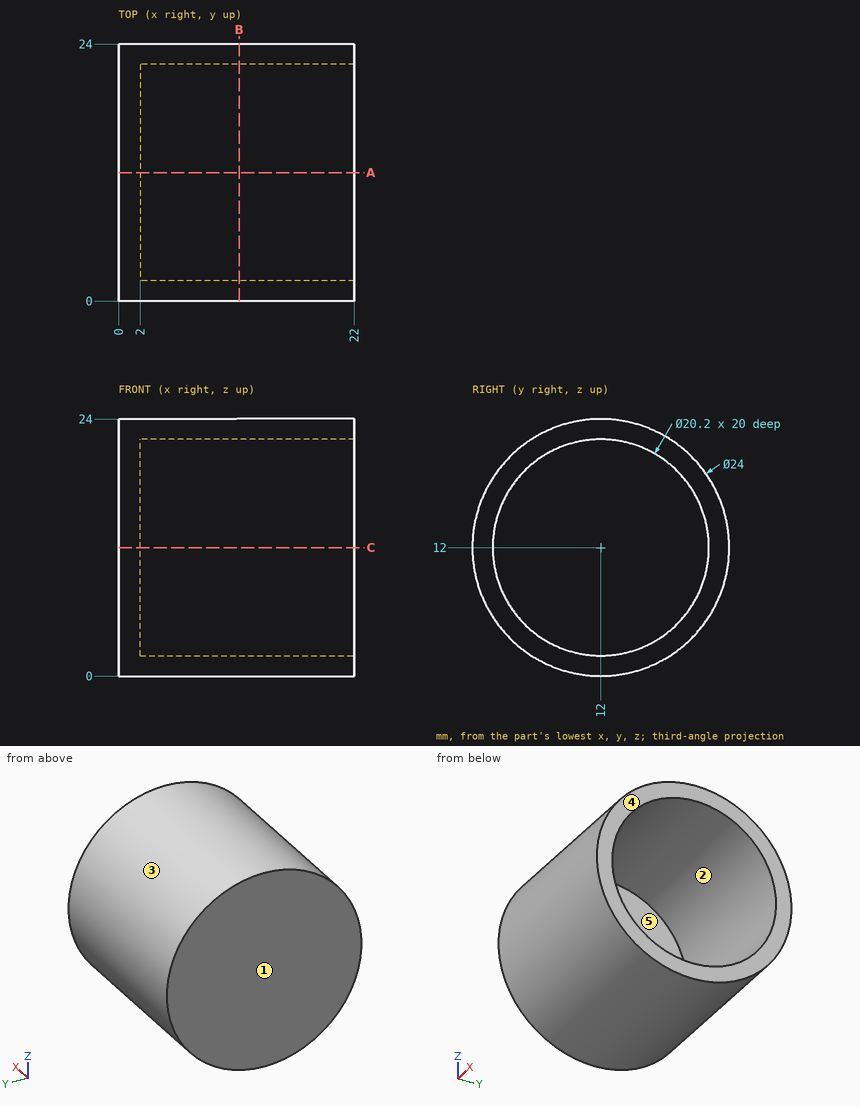
Print and shaded views of the part. All mm, measured from the part's lowest x, y and z. A direction names the side the tool comes from. Coordinates: 2 decimals unless noted, no trailing zeros. Order: outer loops, then holes, each group sorted by start corner. A loop starts at its lowest first (then second) coordinate and runs counter-clockwise, first axis right, second up. Notation, with made-up numbers: (-2, 30.25) - (48, 30.25) arc R13 cw to (48, 50.25) - close; hole circle Ø6 at (55, 46.25). An arc over 180 degrees is marked (long way). Return JSON: item names as keys, results as strings. Group by question number.
Item 1: Pull direction Y, two halves, no side cores. Call the marked faces 3, 4 and 5: pulls with the +Y half, pulls with the -Y half, needs draft (parallel to the pull), parting line crosses it, or undercut.
Item 2: Pin check, flat tips, straight feed: pin 1 (2 mm diameter, centred on x = 16.5, z = 10, fed in from +Y); pin 2 (10 mm diameter, centred on x = 5.5, y = 10, fed in from +Z); pin 3 (2 mm diameter, centred on y = 6, z = 6, fed in from +X); pin 4 (2 mm diameter, centred on x = 4, z = 10, fed in from -Y). Stop position of each tip, or through.
Item 3: Cut at A-A (y = 12). List the corners of the cut face in (x, z).
Item 4: Drill centre lines: probe 1 along Y at (x, z) = (10.75, 12); probe 2 along X at (y, z) = (10, 13.25); probe 3 along Y at (x, z) = (2.5, 9.25). Where is each one in solid material? Low to high. Write a range as from..to.
Item 5: Cut at B-B (x = 11.25). List the corners of the cut face in (y, z).
Item 6: Which spindle directions (+Z, -Z, +X, -X, +Y, -Y) get a long thin tool onto all of the face, cutting with end or side? Do the marked faces 1 and 2. Say none if no direction does.
Check values:
{
 "1": {"face 3": "parting line crosses it", "face 4": "needs draft", "face 5": "undercut"},
 "2": {"pin 1": "stops at y = 23.96", "pin 2": "stops at z = 24", "pin 3": "stops at x = 2", "pin 4": "stops at y = 0.04"},
 "3": {"outline": "(0, 0) - (22, 0) - (22, 1.9) - (2, 1.9) - (2, 22.1) - (22, 22.1) - (22, 24) - (0, 24) - close"},
 "4": {"probe 1": "y = 0..1.9, 22.1..24", "probe 2": "x = 0..2", "probe 3": "y = 0.32..2.28, 21.72..23.68"},
 "5": {"outline": "circle Ø24 at (12, 12); hole circle Ø20.2 at (12, 12)"},
 "6": {"face 1": "+Z, -Z, -X, +Y, -Y", "face 2": "+X"}
}
